Part model, mm, in its own coordinate system. A direction names the side the tool comes from. Give positions to 0.01 mm unless a question says otherwise; leave off trailing zeros. Write each loop counter-clockwise with the first axis right and the second up, starting at its lowest first coordinate (ties: lowest second). Pieces come first, ordered by that corner, then holes. Notation, with made-up numbers: M -38,21 L -26,21 A22 ccw -26,52 Z; hole C 82.25,-33.5 d2. An arc over 180 degrees is marked long. Use CSV: the item, a comma, the result in double quotes. Start each with the question number.
1. Band-saw the part on A-A, the plane x = 0. List the corners of the cut face in (y, z), then the cut area to 3 significant figures.
2. Band-saw the part on B-B, the plane z = 25. Count the separate pieces of the cut face and the enclosed holes in it, then the cut area to 3 significant figures.
3. Drop flat-ended pins along their axis: pin 1 Ø0.6 at (x, y) = (-18, -18.5) entering from +Z; pin 2 Ø5.5 at (x, y) = (-7.75, -6.42) entering from +Z; pin 3 Ø10 at (y, z) = (-19, 15.5) entering from -X. Give the stop position or say it passes through.
4. Mould opens along X. For faces 1 (the face through (-3.303, 25.154, 0.17)), 2 (the face through (-24.295, 0.535, 28.07)) say: pulls with the +X half, pulls with the -X half, needs draft (parallel to the pull), parting line crosses it, or undercut.
5. 3-axis set-ups, long thin cutter, end or side, ignore diameter. For faces 3 (the face through (18.5, 7.1, 1.1)), 4 (the face through (-8.97, -5.31, 4.73)), 5 (the face through (17.8, -17.14, 28.07)): which of +Z, -Z, +X, -X, +Y, -Y reach the whole face in a straight line?
6. Drill centre lines: line 1 along Y through (x, z) = (0, 15); line 2 along X through (y, z) = (7, 1); line 3 along X through (y, z) = (7, 1.2). Where is each one in solid material? Low to high. Write a range as from..to.
7. Band-saw the part on C-C, the plane z = 16.5. List the corners of the cut face in (x, y), then the cut area to 3 significant figures.
from build123d import *

# Parameters (mm, degrees)
SKETCH1_R              = 28.7
SKETCH1_R_2            = 6.15
SKETCH1_R_3            = 1.65
EXTRUDE_506_DEPTH      = 33
SKETCH2_R              = 18.7
CUT_EXTRUDE_685_DEPTH  = 27
CUT_EXTRUDE_START      = -9
SKETCH4_R              = 28.7
SKETCH4_R_2            = 27.7
CUT_EXTRUDE_817_DEPTH  = 9
SKETCH5_R              = 1
CUT_EXTRUDE_1184_DEPTH = 10
CHAMFER1_SIZE          = 3.5
SKETCH_1_R             = 3
CUT_EXTRUDE_1538_DEPTH = 2
CHAMFER_1590_SIZE      = 1.5


with BuildPart() as part:
    # Sketch1 → Extrude 506 (new body)
    with BuildSketch(Plane.XY):
        Circle(SKETCH1_R)
        Circle(SKETCH1_R_2, mode=Mode.SUBTRACT)
        with Locations((15.5, 7)):
            Circle(SKETCH1_R_3, mode=Mode.SUBTRACT)
        with Locations((7.75, -6.423393759)):
            Circle(SKETCH1_R_3, mode=Mode.SUBTRACT)
        with Locations((-7.75, -6.423393759)):
            Circle(SKETCH1_R_3, mode=Mode.SUBTRACT)
        with Locations((-15.5, 7)):
            Circle(SKETCH1_R_3, mode=Mode.SUBTRACT)
        with Locations((-7.75, 20.423393759)):
            Circle(SKETCH1_R_3, mode=Mode.SUBTRACT)
        with Locations((7.75, 20.423393759)):
            Circle(SKETCH1_R_3, mode=Mode.SUBTRACT)
    extrude(amount=EXTRUDE_506_DEPTH)

    # Sketch2 → Cut-Extrude 685 (cut)
    with BuildSketch(Plane.XY.offset(33)):
        with Locations((0, 7)):
            Circle(SKETCH2_R)
    extrude(amount=-CUT_EXTRUDE_685_DEPTH, mode=Mode.SUBTRACT)

    # Sketch4 → Cut-Extrude 817 (cut)
    with BuildSketch(Plane.XY.offset(33).offset(CUT_EXTRUDE_START)):
        Circle(SKETCH4_R)
        Circle(SKETCH4_R_2, mode=Mode.SUBTRACT)
    extrude(amount=CUT_EXTRUDE_817_DEPTH, mode=Mode.SUBTRACT)

    # Sketch5 → Cut-Extrude 1184 (cut)
    with BuildSketch(Plane.XY.offset(33)):
        with Locations((-25.248910365, 0.234574858)):
            Circle(SKETCH5_R)
        with Locations((-17.587461053, -18.117497446)):
            Circle(SKETCH5_R)
        with Locations(Location((17.587461053, -18.117497446, 0), (0, 0, 180))):
            Circle(SKETCH5_R)
        with Locations(Location((25.248910365, 0.234574858, 0), (0, 0, 180))):
            Circle(SKETCH5_R)
        with Locations((-16.85427288, 18.801488922)):
            Circle(SKETCH5_R)
        with Locations(Location((16.85427288, 18.801488922, 0), (0, 0, 180))):
            Circle(SKETCH5_R)
        with Locations((0, -25.25)):
            Circle(SKETCH5_R)
    extrude(amount=-CUT_EXTRUDE_1184_DEPTH, mode=Mode.SUBTRACT)

    # Chamfer1
    chamfer1_edges = [part.edges().sort_by_distance(p)[0] for p in [
        (-28.7, 0, 0),
    ]]
    chamfer(chamfer1_edges, length=CHAMFER1_SIZE)

    # Эскиз1 → Cut-Extrude 1538 (cut)
    with BuildSketch(Plane(origin=(0, 0, 0), x_dir=(-1, 0, 0), z_dir=(0, 0, -1))):
        with Locations((-7.75, 20.423393759)):
            Circle(SKETCH_1_R)
        with Locations((7.75, 20.423393759)):
            Circle(SKETCH_1_R)
        with Locations((15.5, 7)):
            Circle(SKETCH_1_R)
        with Locations((7.75, -6.423393759)):
            Circle(SKETCH_1_R)
        with Locations((-7.75, -6.423393759)):
            Circle(SKETCH_1_R)
        with Locations((-15.5, 7)):
            Circle(SKETCH_1_R)
    extrude(amount=-CUT_EXTRUDE_1538_DEPTH, mode=Mode.SUBTRACT)

    # Chamfer 1590
    # the kernel refuses this chamfer: 1.5 mm, written as the material it takes off along each edge
    with BuildSketch(Plane(origin=(15.5, 7, 2), x_dir=(1, 0, 0), z_dir=(0, 1, 0))) as chamfer_1590_piece_1_section:
        Polygon((1.65 + CHAMFER_1590_SIZE, 0), (1.65, -CHAMFER_1590_SIZE), (1.65, 0), align=None)
    chamfer_1590_piece_1 = revolve(axis=Axis((15.5, 7, 2), (0, 0, -1)), mode=Mode.PRIVATE)
    chamfer_1590_piece_1 = chamfer_1590_piece_1 & Plane(origin=(15.5, 7, 2.828305934), x_dir=(-1, 0, 0), z_dir=(0, 0, -1)) * Cylinder(3, 13, mode=Mode.PRIVATE)
    add(chamfer_1590_piece_1, mode=Mode.SUBTRACT)
    with BuildSketch(Plane(origin=(7.75, -6.423393759, 2), x_dir=(1, 0, 0), z_dir=(0, 1, 0))) as chamfer_1590_piece_2_section:
        Polygon((1.65 + CHAMFER_1590_SIZE, 0), (1.65, -CHAMFER_1590_SIZE), (1.65, 0), align=None)
    chamfer_1590_piece_2 = revolve(axis=Axis((7.75, -6.423393759, 2), (0, 0, -1)), mode=Mode.PRIVATE)
    chamfer_1590_piece_2 = chamfer_1590_piece_2 & Plane(origin=(7.75, -6.423393759, 2.828305934), x_dir=(-1, 0, 0), z_dir=(0, 0, -1)) * Cylinder(3, 13, mode=Mode.PRIVATE)
    add(chamfer_1590_piece_2, mode=Mode.SUBTRACT)
    with BuildSketch(Plane(origin=(-7.75, -6.423393759, 2), x_dir=(1, 0, 0), z_dir=(0, 1, 0))) as chamfer_1590_piece_3_section:
        Polygon((1.65 + CHAMFER_1590_SIZE, 0), (1.65, -CHAMFER_1590_SIZE), (1.65, 0), align=None)
    chamfer_1590_piece_3 = revolve(axis=Axis((-7.75, -6.423393759, 2), (0, 0, -1)), mode=Mode.PRIVATE)
    chamfer_1590_piece_3 = chamfer_1590_piece_3 & Plane(origin=(-7.75, -6.423393759, 2.828305934), x_dir=(-1, 0, 0), z_dir=(0, 0, -1)) * Cylinder(3, 13, mode=Mode.PRIVATE)
    add(chamfer_1590_piece_3, mode=Mode.SUBTRACT)
    with BuildSketch(Plane(origin=(-15.5, 7, 2), x_dir=(1, 0, 0), z_dir=(0, 1, 0))) as chamfer_1590_piece_4_section:
        Polygon((1.65 + CHAMFER_1590_SIZE, 0), (1.65, -CHAMFER_1590_SIZE), (1.65, 0), align=None)
    chamfer_1590_piece_4 = revolve(axis=Axis((-15.5, 7, 2), (0, 0, -1)), mode=Mode.PRIVATE)
    chamfer_1590_piece_4 = chamfer_1590_piece_4 & Plane(origin=(-15.5, 7, 2.828305934), x_dir=(-1, 0, 0), z_dir=(0, 0, -1)) * Cylinder(3, 13, mode=Mode.PRIVATE)
    add(chamfer_1590_piece_4, mode=Mode.SUBTRACT)
    with BuildSketch(Plane(origin=(-7.75, 20.423393759, 2), x_dir=(1, 0, 0), z_dir=(0, 1, 0))) as chamfer_1590_piece_5_section:
        Polygon((1.65 + CHAMFER_1590_SIZE, 0), (1.65, -CHAMFER_1590_SIZE), (1.65, 0), align=None)
    chamfer_1590_piece_5 = revolve(axis=Axis((-7.75, 20.423393759, 2), (0, 0, -1)), mode=Mode.PRIVATE)
    chamfer_1590_piece_5 = chamfer_1590_piece_5 & Plane(origin=(-7.75, 20.423393759, 2.828305934), x_dir=(-1, 0, 0), z_dir=(0, 0, -1)) * Cylinder(3, 13, mode=Mode.PRIVATE)
    add(chamfer_1590_piece_5, mode=Mode.SUBTRACT)
    with BuildSketch(Plane(origin=(7.75, 20.423393759, 2), x_dir=(1, 0, 0), z_dir=(0, 1, 0))) as chamfer_1590_piece_6_section:
        Polygon((1.65 + CHAMFER_1590_SIZE, 0), (1.65, -CHAMFER_1590_SIZE), (1.65, 0), align=None)
    chamfer_1590_piece_6 = revolve(axis=Axis((7.75, 20.423393759, 2), (0, 0, -1)), mode=Mode.PRIVATE)
    chamfer_1590_piece_6 = chamfer_1590_piece_6 & Plane(origin=(7.75, 20.423393759, 2.828305934), x_dir=(-1, 0, 0), z_dir=(0, 0, -1)) * Cylinder(3, 13, mode=Mode.PRIVATE)
    add(chamfer_1590_piece_6, mode=Mode.SUBTRACT)


solid = part.part
Output:
1,outline,"M -28.7,3.5 L -25.2,0 L -6.15,0 L -6.15,6 L -11.7,6 L -11.7,33 L -24.25,33 L -24.25,23 L -26.25,23 L -26.25,33 L -27.7,33 L -27.7,24 L -28.7,24 Z; M 6.15,0 L 25.2,0 L 28.7,3.5 L 28.7,24 L 27.7,24 L 27.7,33 L 25.7,33 L 25.7,6 L 6.15,6 Z"
1,area,"760 mm²"
2,separate pieces,"1"
2,enclosed holes,"8"
2,area,"1,290 mm²"
3,pin 1,"stops at z = 23"
3,pin 2,"stops at z = 6"
3,pin 3,"stops at x = -25.05"
4,face 1,"parting line crosses it"
4,face 2,"undercut"
5,face 3,"-Z"
5,face 4,"+Z, -Z"
5,face 5,"+Z"
6,line 1,"y = -28.7..-11.7, 25.7..28.7"
6,line 2,"x = -25.25..-18.5, -12.5..12.5, 18.5..25.25"
6,line 3,"x = -25.46..-18.5, -12.5..12.5, 18.5..25.46"
7,outline,"C 0,0 d57.4; hole C 0,7 d37.4"
7,area,"1,490 mm²"
